Geometry check sheet. Reference: the model listing, model coordinates, mm. Give positions to 0.01 mm unless a question says otherwise; leave off trailing zeros. Order: outer loops, then holes, each group sorted by start corner. A loop starts at its lowest first (then second) coordinate and runs counter-clockwise, first axis right, second up. Notation, with made-up numbers: M 50.25,-5.5 L 85.25,-5.5 A25 cw 85.25,9.5 Z; hole C 30.5,-2 d2. An arc over 180 degrees is marked long. Answer as CSV lines item,"result". Start each with the question number.
Q1. Thickness scan on line 1 (X direction, y = -16.5, z = 21.5); line 2 (X direction, y = -13, z = 31.5); line 3 (X direction, y = -12, z = 30). Record the ranges inside material, lowest first.
Q2. Section check B-B, the plane y = -16. Record the boundary of the cut face in (x, z) (3 decimals), then the cut area to 3 significant figures.
Q3. Section check C-C, the plane z = 40. Record the boundary of the cut face in (x, y).
Q4. Mould release check, pull along X, two halves, no side actions. Record for faces 1 (the cylindrical face through (119.534, -9.392, 36.186)), 2 (the cylindrical face through (125.863, -9.658, 40.464)), 3 (the flat face through (11, -9, 43.18)): +X half, -X half, draft (parallel to the pull), parting line (faces both ways), or undercut.
Q5. Section check A-A, the plane z = 21.59. Record the boundary of the cut face in (x, y).
```python
from build123d import *

# Parameters (mm, degrees)
F1_DEPTH = 19.05
F2_D     = 10.0838
F3_R     = 9.525
F5_D     = 5.1054


with BuildPart() as f1:
    # F0 (on Front) → F1 (new body)
    with BuildSketch(Plane.XZ):
        with BuildLine():
            Line((128.7268799004, 43.18), (-99.8731200996, 43.18))
            ThreePointArc((-99.8731200996, 43.18), (-121.4631200996, 21.59), (-99.8731200996, 0))
            Line((-99.8731200996, 0), (128.7268799004, 0))
            Line((128.7268799004, 0), (128.7268799004, 43.18))
        make_face()
    extrude(amount=F1_DEPTH)

    # F2 (through all)
    with Locations(Plane(origin=(0, 0, 0), x_dir=(1, 0, 0), z_dir=(0, 1, 0))):
        with Locations((-99.8731200996, -21.59)):
            Hole(F2_D / 2)

    # F3
    f3_edges = [f1.edges().sort_by_distance(p)[0] for p in [
        (128.72688, -9.525, 43.18),
    ]]
    fillet(f3_edges, radius=F3_R)

    # F5 (through all)
    with Locations(Plane.XZ.offset(19.05)):
        with Locations((119.2018799004, 33.655), (119.2018799004, 9.525)):
            Hole(F5_D / 2)


solid = f1.part
```
Answer block:
1,line 1,"x = -121.46 to -104.91, -94.83 to 128.73"
1,line 2,"x = -119.05 to 117.83, 120.57 to 128.73"
1,line 3,"x = -119.76 to 128.73"
2,outline,"M -99.873,0 L 128.727,0 L 128.727,33.655 A9.525 ccw 119.202,43.18 L -99.873,43.18 A21.59 ccw Z; hole C -99.873,21.59 d10.084; hole C 119.202,9.525 d5.105; hole C 119.202,33.655 d5.105"
2,area,"10,500 mm2"
3,outline,"M -111.15,-19.05 L 126.31,-19.05 L 126.31,0 L -111.15,0 Z"
4,face 1,"undercut"
4,face 2,"+X half"
4,face 3,"draft"
5,outline,"M -121.46,-19.05 L -104.92,-19.05 L -104.92,0 L -121.46,0 Z; M -94.83,-19.05 L 128.73,-19.05 L 128.73,0 L -94.83,0 Z"
